Read the model definition and answer for the solid it produces. Units are mm, in the model's axes. A direction names the side the tool comes from. Coordinates: 2 decimals unless noted, no trailing zeros. Loops run counter-clockwise (first coordinate to the right, second up) from the corner with the lowest first, then second, coordinate; pieces in that order, holes last. Notation, with made-up numbers: (-26.5, 7.25) -> (-16.5, 7.25) arc R20 cw to (-16.5, 22.25) -> close; hole circle Ø6 at (-20.5, -22.5). An arc over 180 degrees is marked (long way). Answer as a JSON object with one key per item and string values. Group by question number.
Q1. The part is cut by section A-A on y = 15.75. Write down the section's boundary in (x, z), and give its area (3 significant figures).
Q2. Straight lines are drawn through the part: line 1 along X through (y, z) = (7, 0); line 2 along Y through (x, z) = (5.25, 5); line 3 along X through (y, z) = (15, -2.25). For each, find the intervals that lie inside material, in ascending order. Write a range as [from, to].
Q3. The part is cut by section C-C on y = 9.25. Write down the section's boundary in (x, z), and give its area (3 significant figures).
Q4. The part is cut by section D-D on y = 4.25. Write down the section's boundary in (x, z), and give its area (3 significant figures).
Q5. The part is cut by section B-B on x = 0. Write down the section's boundary in (y, z), and give its area (3 significant figures).
Q6. Each of these flat-tipped pins is pushed along its axis until it touches: P1, Ø2, axis at x = -1.5, y = 13.5, coming from the -Z side; P2, Ø1.5, axis at x = -6, y = 7.5, coming from the -Z side; P3, Ø1, axis at x = 7, y = 12.5, coming from the +Z side. Where does it stop, or does it pass through?
Q7. For faces 4 (the flat face through (0, 17, -7)), 5 (the flat face through (-7.3, 9, 0)), 6 (the flat face through (-5.6, 13.6, -3.3)), determine the directions among +Z, -Z, +X, -X, +Y, -Y from which every point of the face is accessible in a straight line to the end or side of a thin tool.
Q8. Determine the mould class of faces 1 (the flat face through (-6, 4, 4)), 2 (the flat face through (0, 14, 6.5)), 3 (the flat face through (3, 10.2, -3)) for opening direction Y: released by +Y, released by -Y, zero draft, split by the parting line, or undercut.
from build123d import *

# Parameters (mm, degrees)
SKETCH1_R           = 9
BOSS_EXTRUDE1_DEPTH = 4
SKETCH2_R           = 7
BOSS_EXTRUDE2_DEPTH = 5
SKETCH4_R           = 9
BOSS_EXTRUDE3_DEPTH = 8
FILLET1_R           = 1
FILLET2_R           = 1
SKETCH5_R           = 4
CUT_EXTRUDE1_DEPTH  = 18
CUT_EXTRUDE2_DEPTH  = 6.8


with BuildPart() as part:
    # Sketch1 → Boss-Extrude1 (new body)
    with BuildSketch(Plane(origin=(0, 0, 0), x_dir=(1, 0, 0), z_dir=(0, 1, 0))):
        with Locations(Location((0, 0, 0), (0, 0, 270))):
            Circle(SKETCH1_R)
    extrude(amount=BOSS_EXTRUDE1_DEPTH)

    # Sketch2 → Boss-Extrude2 (add)
    with BuildSketch(Plane(origin=(0, 4, 0), x_dir=(1, 0, 0), z_dir=(0, 1, 0))):
        with Locations(Location((0, 0, 0), (0, 0, 270))):
            Circle(SKETCH2_R)
    extrude(amount=BOSS_EXTRUDE2_DEPTH)

    # Sketch4 → Boss-Extrude3 (add)
    with BuildSketch(Plane(origin=(0, 9, 0), x_dir=(1, 0, 0), z_dir=(0, 1, 0))):
        with Locations(Location((0, 0, 0), (0, 0, 270))):
            Circle(SKETCH4_R)
    extrude(amount=BOSS_EXTRUDE3_DEPTH)

    # Fillet1
    fillet1_edges = [part.edges().sort_by_distance(p)[0] for p in [
        (0, 17, -9),
    ]]
    fillet(fillet1_edges, radius=FILLET1_R)

    # Fillet2
    fillet2_edges = [part.edges().sort_by_distance(p)[0] for p in [
        (0, 4, -9),
    ]]
    fillet(fillet2_edges, radius=FILLET2_R)

    # Sketch5 → Cut-Extrude1 (cut)
    with BuildSketch(Plane.XZ):
        with Locations(Location((0, 0, 0), (0, 0, 270))):
            Circle(SKETCH5_R)
    extrude(amount=-CUT_EXTRUDE1_DEPTH, mode=Mode.SUBTRACT)

    # Sketch6 → Cut-Extrude2 (cut)
    with BuildSketch(Plane(origin=(0, 17, 0), x_dir=(1, 0, 0), z_dir=(0, 1, 0))):
        Polygon((-7.505553499, 0), (-3.75277675, -6.5), (3.75277675, -6.5), (7.505553499, 0), (3.75277675, 6.5), (-3.75277675, 6.5), align=None)
    extrude(amount=-CUT_EXTRUDE2_DEPTH, mode=Mode.SUBTRACT)


solid = part.part
Final values:
{
 "1": {"outline": "circle Ø18 at (0, 0); hole (-7.51, 0) -> (-3.75, -6.5) -> (3.75, -6.5) -> (7.51, 0) -> (3.75, 6.5) -> (-3.75, 6.5) -> close", "area": "108 mm2"},
 "2": {"line 1": "x = [-7, -4], [4, 7]", "line 2": "y = [0, 4], [9, 17]", "line 3": "x = [-8.71, -6.21], [6.21, 8.71]"},
 "3": {"outline": "circle Ø18 at (0, 0); hole circle Ø8 at (0, 0)", "area": "204 mm2"},
 "4": {"outline": "circle Ø14 at (0, 0); hole circle Ø8 at (0, 0)", "area": "104 mm2"},
 "5": {"outline": "(0, -9) -> (3, -9) arc R1 ccw to (4, -8) -> (4, -7) -> (9, -7) -> (9, -9) -> (16, -9) arc R1 ccw to (17, -8) -> (17, -6.5) -> (10.2, -6.5) -> (10.2, -4) -> (0, -4) -> close; (0, 4) -> (10.2, 4) -> (10.2, 6.5) -> (17, 6.5) -> (17, 8) arc R1 ccw to (16, 9) -> (9, 9) -> (9, 7) -> (4, 7) -> (4, 8) arc R1 ccw to (3, 9) -> (0, 9) -> close", "area": "115 mm2"},
 "6": {"P1": "stops at z = -8.99", "P2": "stops at z = -4.63", "P3": "stops at z = 6.22"},
 "7": {"face 4": "+Z, -Z, +X, -X, +Y", "face 5": "none", "face 6": "+Y"},
 "8": {"face 1": "undercut", "face 2": "zero draft", "face 3": "released by +Y"}
}
